Source: CAD feature listing. Evaluate the final solid. Frame: model axes, mm. Face numbers are marked on the shaded views. A direction names the side the tool comes from. Give positions to 0.01 mm unless a question says otherwise; leave off trailing zeros. Write each loop counter-clockwise with the first axis right and the second up, starting at its lowest first coordinate (ties: lowest second). Pieces come first, ordered by that corner, then holes.
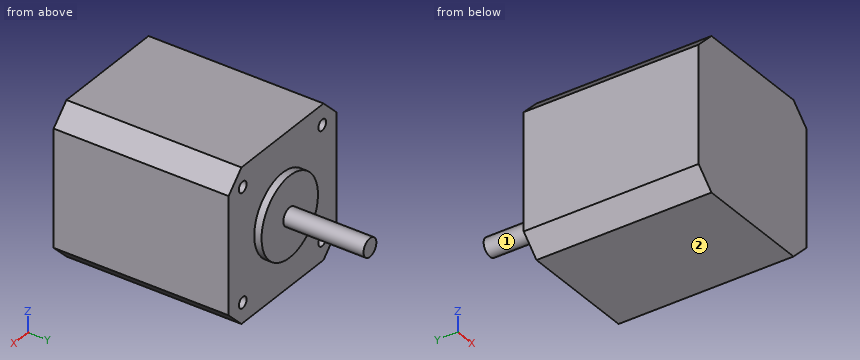
```python
from build123d import *

# Parameters (mm, degrees)
SKETCH1_W           = 42
SKETCH1_H           = 42
BOSS_EXTRUDE1_DEPTH = 48
CHAMFER1_SIZE       = 5
SKETCH2_R           = 1.5
CUT_EXTRUDE1_DEPTH  = 4.5
SKETCH3_R           = 11
BOSS_EXTRUDE2_DEPTH = 2
SKETCH4_R           = 2.5
BOSS_EXTRUDE3_DEPTH = 22


with BuildPart() as part:
    # Sketch1 → Boss-Extrude1 (new body)
    with BuildSketch(Plane(origin=(0, 0, 0), x_dir=(1, 0, 0), z_dir=(0, 1, 0))):
        with Locations((21, 21)):
            Rectangle(SKETCH1_W, SKETCH1_H)
    extrude(amount=BOSS_EXTRUDE1_DEPTH)

    # Chamfer1
    chamfer1_edges = [part.edges().sort_by_distance(p)[0] for p in [
        (0, 24, -42),
        (42, 24, -42),
        (42, 24, 0),
        (0, 24, 0),
    ]]
    chamfer(chamfer1_edges, length=CHAMFER1_SIZE)

    # Sketch2 → Cut-Extrude1 (cut)
    with BuildSketch(Plane(origin=(0, 48, 0), x_dir=(1, 0, 0), z_dir=(0, 1, 0))):
        with Locations(Location((5.5, 36.5, 0), (0, 0, 270))):
            Circle(SKETCH2_R)
        with Locations(Location((36.5, 36.5, 0), (0, 0, 270))):
            Circle(SKETCH2_R)
        with Locations(Location((5.5, 5.5, 0), (0, 0, 270))):
            Circle(SKETCH2_R)
        with Locations(Location((36.5, 5.5, 0), (0, 0, 270))):
            Circle(SKETCH2_R)
    extrude(amount=-CUT_EXTRUDE1_DEPTH, mode=Mode.SUBTRACT)

    # Sketch3 → Boss-Extrude2 (add)
    with BuildSketch(Plane(origin=(0, 48, 0), x_dir=(1, 0, 0), z_dir=(0, 1, 0))):
        with Locations(Location((21, 21, 0), (0, 0, 90))):
            Circle(SKETCH3_R)
    extrude(amount=BOSS_EXTRUDE2_DEPTH)

    # Sketch4 → Boss-Extrude3 (add)
    with BuildSketch(Plane(origin=(0, 50, 0), x_dir=(1, 0, 0), z_dir=(0, 1, 0))):
        with Locations(Location((21, 21, 0), (0, 0, 270))):
            Circle(SKETCH4_R)
    extrude(amount=BOSS_EXTRUDE3_DEPTH)


solid = part.part
```
1. Access query for the marked faces 1 and 2. Directions: +Z, -Z, +X, -X, +Y, -Y. A direction counts if a zero-diameter tool reaches every point of the face in a straight line with its end or side. Return the directions, or none.
2. Section query C-C (z = -21). Return loops of the section in (x, y), plus the area to 3 significant figures.
3. Section query D-D (x = 21). Return loops of the section in (y, z), plus the area to 3 significant figures.
4. Line query: probe 1 along X at (y, z) = (45.1, -36.5); probe 2 along Y at (x, z) = (15.5, -11); probe 3 along X at (y, z) = (45, -36). Output: solid intervals per line, ascending.
5. Section query B-B (y = 29.5). Return loops of the section in (x, z), plus the area to 3 significant figures.
6. Pin query (flat end, axial travel): P1, Ø3.5, axis at x = 37, z = -5.5, coming from the +Y side; P2, Ø12, axis at y = 59, z = -11, coming from the +X side; P3, Ø8, axis at x = 16, y = 63, coming from the -Z side. Return the tip coordinate at first contact, or that it passes through.
7. Section query A-A (y = 44.5). Return loops of the section in (x, z).
The answers:
1. face 1: +Y
1. face 2: -Z, +X, -X, +Y, -Y
2. outline: (0, 0) - (42, 0) - (42, 48) - (32, 48) - (32, 50) - (23.5, 50) - (23.5, 72) - (18.5, 72) - (18.5, 50) - (10, 50) - (10, 48) - (0, 48) - close
2. area: 2,170 mm2
3. outline: (0, -42) - (48, -42) - (48, -32) - (50, -32) - (50, -23.5) - (72, -23.5) - (72, -18.5) - (50, -18.5) - (50, -10) - (48, -10) - (48, 0) - (0, 0) - close
3. area: 2,170 mm2
4. probe 1: x = 0 to 4, 7 to 35, 38 to 42
4. probe 2: y = 0 to 48
4. probe 3: x = 0 to 4.09, 6.91 to 35.09, 37.91 to 42
5. outline: (0, -37) - (5, -42) - (37, -42) - (42, -37) - (42, -5) - (37, 0) - (5, 0) - (0, -5) - close
5. area: 1,710 mm2
6. P1: stops at y = 48
6. P2: passes through
6. P3: stops at z = -23.29
7. outline: (0, -37) - (5, -42) - (37, -42) - (42, -37) - (42, -5) - (37, 0) - (5, 0) - (0, -5) - close; hole circle Ø3 at (5.5, -36.5); hole circle Ø3 at (5.5, -5.5); hole circle Ø3 at (36.5, -36.5); hole circle Ø3 at (36.5, -5.5)
